Autodesk Inventor part; units mm, degrees
ref_plane "YZ Plane" through (0, 0, 0) normal (1, 0, 0) x (0, 1, 0)
ref_plane "XZ Plane" through (0, 0, 0) normal (0, 1, 0) x (-1, 0, 0)
ref_plane "XY Plane" through (0, 0, 0) normal (0, 0, 1) x (1, 0, 0)
sketch "Sketch1" plane through (0, 0, 0) normal (0, 1, 0) x (-1, 0, 0)
  circle A0 centre (0, 0) radius 9.8425
  circle A1 centre (0, 0) radius 5.08
  dimension "d0" = 19.685
  dimension "d1" = 10.16
extrude "Extrusion1" add sketch "Sketch1" along normal blind 44.45
sketch "Sketch2" plane through (0, 0, 0) normal (0, -1, 0) x (1, 0, 0)
  circle A0 centre (0, 0) radius 9.8425
  line L0 (4.0695, 16.6582) -> (16.4611, -4.8048)
  line L1 (12.3917, -11.8533) -> (-12.3917, -11.8533)
  line L2 (-16.4611, -4.8048) -> (-4.0695, 16.6582)
  arc A1 (4.0695, 16.6582) -> (-4.0695, 16.6582) centre (0, 14.3087) ccw
  arc A2 (-16.4611, -4.8048) -> (-12.3917, -11.8533) centre (-12.3917, -7.1543) ccw
  arc A3 (12.3917, -11.8533) -> (16.4611, -4.8048) centre (12.3917, -7.1543) ccw
  circle A4 centre (0, 0) radius 5.08
  circle A5 centre (0, 0) radius 5.08
  point P0 (0, 23.7067)
  point P1 (20.5306, -11.8533)
  point P2 (-20.5306, -11.8533)
  dimension "d4" = 35.56
  dimension "d5" = 35.56
  dimension "d6" = 4.699
  dimension "d7" = 4.699
  dimension "d8" = 4.699
extrude "Extrusion2" add sketch "Sketch2" along normal blind 5.08 contours A0 | L0 A3 L1 A2 L2 A1
sketch "Sketch3" plane through (0, -5.08, 0) normal (0, -1, 0) x (1, 0, 0)
  arc A0 (4.0695, 16.6582) -> (-4.0695, 16.6582) centre (0, 14.3087) ccw
  arc A1 (-16.4611, -4.8048) -> (-12.3917, -11.8533) centre (-12.3917, -7.1543) ccw
  arc A2 (12.3917, -11.8533) -> (16.4611, -4.8048) centre (12.3917, -7.1543) ccw
  circle A3 centre (0, 14.3087) radius 2.54
  circle A4 centre (12.3917, -7.1543) radius 2.54
  circle A5 centre (-12.3917, -7.1543) radius 2.54
  dimension "d11" = 5.08
  dimension "d12" = 5.08
  dimension "d13" = 5.08
extrude "Extrusion3" cut sketch "Sketch3" against normal blind 5.08
properties part number "ScrewShaft"
The listing builds one solid part. Answer for the finished solid, in the listing's coordinates (mm). A direction names the side the tool comes from. Round coordinates to 2 decimals unless told otherwise and drop trailing zeros. Order: outer loops, then holes, each group sorted by start corner. A loop starts at its lowest first (then second) coordinate and runs counter-clockwise, first axis right, second up. Notation, with made-up numbers: (-24.75, 60) - (3.25, 60) arc R14 cw to (3.25, 85) - close; hole circle Ø6 at (57, 22). An arc over 180 degrees is marked (long way). Write item = value, one per line. Start each with the question number.
1) Given pin 1 (3 mm diameter, centred on y = 30.5, z = -6.5, fed in from -X); pin 2 (5 mm diameter, centred on x = 2, y = 36, fed in from +Z); pin 3 (1 mm diameter, centred on x = 7, y = 4.5, fed in from +Z), each flat-ended and moving along its own axis, determine where each tip first touches the part or whether it passes through.
2) For faces 4 (the flat face through (-9, 0, 5)), 5 (the flat face through (0, -3, -11.853)), determine the directions among +Z, -Z, +X, -X, +Y, -Y from which every point of the face is accessible in a straight line to the end or side of a thin tool.
3) Section A-A, the plane x = 0 is taken. Write down the section's boundary in (y, z), plus the area to 3 significant figures.
4) Section B-B, the plane y = 4.5 is taken. Write down the section's boundary in (x, z) (1 decimal), plus the area to 3 significant figures.
5) Section C-C, the plane z = 13 is taken. Write down the section's boundary in (x, y).
6) For a pull along Z with two mould halves and no side action, classify faces 1 (the cylindrical face through (1.365, -2.576, 16.45)), 2 (the cylindrical face through (16.495, -2.504, -9.444)), 3 (the cylindrical face through (-0.069, -2.504, 19.007)) as released by +Z, released by -Z, zero draft, split by the parting line, or undercut.
7) Section D-D, the plane x = -7 is taken. Write down the section's boundary in (y, z).
8) Straight lines are drawn through the part: L1, parallel to Z at x = 0, y = 34; L2, parallel to Z at x = -1.5, y = 24.5; L3, parallel to X at y = 10.5, z = 0.5. For each, find the intervals that lie inside material, in ascending order.
Results list:
q1.pin_1 = -8.48
q1.pin_2 = 9.84
q1.pin_3 = 7.39
q2.face_4 = +Y
q2.face_5 = -Z, +X, -X, +Y, -Y
q3.outline = (-5.08, -11.85) - (0, -11.85) - (0, -9.84) - (44.45, -9.84) - (44.45, -5.08) - (-5.08, -5.08) - close; (-5.08, 5.08) - (44.45, 5.08) - (44.45, 9.84) - (0, 9.84) - (0, 11.77) - (-5.08, 11.77) - close; (-5.08, 16.85) - (0, 16.85) - (0, 19.01) - (-5.08, 19.01) - close
q3.area = 503 mm^2
q4.outline = circle Ø19.7 at (0, 0); hole circle Ø10.2 at (0, 0)
q4.area = 223 mm^2
q5.outline = (-6.18, -5.08) - (-2.18, -5.08) - (-2.18, 0) - (-6.18, 0) - close; (2.18, -5.08) - (6.18, -5.08) - (6.18, 0) - (2.18, 0) - close
q6.face_1 = undercut
q6.face_2 = split by the parting line
q6.face_3 = released by +Z
q7.outline = (-5.08, -11.85) - (0, -11.85) - (0, -6.92) - (44.45, -6.92) - (44.45, 6.92) - (0, 6.92) - (0, 11.58) - (-5.08, 11.58) - close
q8.L1 = -9.84 to -5.08, 5.08 to 9.84
q8.L2 = -9.73 to -4.85, 4.85 to 9.73
q8.L3 = -9.83 to -5.06, 5.06 to 9.83
